Geometry check sheet. Reference: the model listing, model coordinates, mm. A direction names the side the tool comes from. Coordinates: 2 decimals unless noted, no trailing zeros. Write each loop counter-clockwise with the first axis right and the second up, starting at its lowest first coordinate (ties: lowest second). Pieces come first, ordered by that corner, then holes. Notation, with made-up numbers: M 47.5,-10.75 L 71.5,-10.75 A20 cw 71.5,25.25 Z; hole C 37,72.25 d2. An arc over 180 degrees is marked long. Put each result on its own line as item: value. Start each with the question number.
1) Cross-section at A-A on y = 0. Record the cut outline in (x, z), plus the area to 3 significant figures.
2) Cross-section at C-C on x = 21. Record the cut outline in (y, z).
3) Mould release check, pull along Y, two halves, no side actions. Record for faces 1 (the flat face through (0, 0, 0)), 2 (the cylindrical face through (12.86, 3.16, -7.62)), 3 (the flat face through (3, 0, 0)), 4 (the cylindrical face through (12.86, 10.006, 2.222)): released by +Y, released by -Y, zero draft, split by the parting line, or undercut.
4) Gauge pin test, flat ends, axial feed: pin 1 (2 mm diameter, centred on x = 19.5, z = -7, fed in from +Y); pin 2 (8 mm diameter, centred on x = 3, z = -12, fed in from -Y); pin 3 (12 mm diameter, centred on x = 17.5, z = 15, fed in from +Y). Record the tip position at first contact, or that the pin passes through.
5) Scan lines: line 1 along Y through (x, z) = (8.5, 0); line 2 along X through (y, z) = (11, 4); line 3 along Z through (x, y) = (20.25, -1). Record each from-to range of solid material in increasing order.
6) Cross-section at D-D on y = -13.5. Record the cut outline in (x, z).
7) Set-up check for faces 5 (the cylindrical face through (1.479, 10.382, 19.961)), 6 (the flat face through (3, 5, -10)): record each of +Z, -Z, +X, -X, +Y, -Y from which the full face is reachable in a straight line by a thin tool's end or side.
Autodesk Inventor part; units mm, degrees
ref_plane "YZ Plane" through (0, 0, 0) normal (1, 0, 0) x (0, 1, 0)
ref_plane "XZ Plane" through (0, 0, 0) normal (0, 1, 0) x (-1, 0, 0)
ref_plane "XY Plane" through (0, 0, 0) normal (0, 0, 1) x (1, 0, 0)
sketch "Sketch1" plane through (0, 0, 0) normal (1, 0, 0) x (0, 1, 0)
  circle A0 centre (0, 0) radius 22.5
  dimension "d0" = 45
extrude "Extrusion1" add sketch "Sketch1" along normal blind 3
sketch "Sketch2" plane through (3, 0, 0) normal (1, 0, 0) x (0, 0, -1)
  circle A0 centre (0, 0) radius 10.25
  circle A1 centre (0, 0) radius 8.25
  dimension "d3" = 20.5
  dimension "d4" = 16.5
extrude "Extrusion2" add sketch "Sketch2" along normal blind 20
properties part number "Leg EndCap - ForPoolNoodle" material "ABS Plastic"
Answer key:
1. outline: M 0,-22.5 L 3,-22.5 L 3,-10.25 L 23,-10.25 L 23,-8.25 L 3,-8.25 L 3,8.25 L 23,8.25 L 23,10.25 L 3,10.25 L 3,22.5 L 0,22.5 Z
1. area: 215 mm²
2. outline: C 0,0 d20.5; hole C 0,0 d16.5
3. face 1: zero draft
3. face 2: undercut
3. face 3: undercut
3. face 4: split by the parting line
4. pin 1: stops at y = 8.31
4. pin 2: stops at y = -21.03
4. pin 3: stops at y = 4.91
5. line 1: y = -10.25 to -8.25, 8.25 to 10.25
5. line 2: x = 0 to 3
5. line 3: z = -10.2 to -8.19, 8.19 to 10.2
6. outline: M 0,-18 L 3,-18 L 3,18 L 0,18 Z
7. face 5: +X, -X
7. face 6: +X
